CAD build for the part. Positions are in the model's coordinates, mm. A direction names the side the tool comes from. Round coordinates to 2 decimals unless told otherwise and drop trailing zeros. Order: outer loops, then holes, each group sorted by start corner. A loop starts at its lowest first (then second) coordinate and runs counter-clockwise, first axis right, second up. Notation, with made-up numbers: M 28,-13 L 44,-13 A15 ccw 44,10 Z; hole C 7.25,85 d2. An arc over 180 degrees is marked long. Answer as CSV lines item,"result". Start each with the question number.
```python
from build123d import *

# Parameters (mm, degrees)
SKETCH_1_R          = 1.6
SKETCH_1_R_2        = 2.1
EXTRUDE_2_DEPTH     = 3
SKETCH_2_R          = 2.1
CUT_EXTRUDE_1_DEPTH = 3
FILLET_1_R          = 3
CUT_EXTRUDE_2_DEPTH = 281.258651654


with BuildPart() as part:
    # 草图1 → 凸台-拉伸2 (new body)
    with BuildSketch(Plane.XY):
        Polygon((20.192307692, -5), (109.041451884, -5), (135.57179677, -50.951905284), (275.57179677, -50.951905284), (275.57179677, 31.048094716), (260.57179677, 31.048094716), (260.57179677, -38.951905284), (142.5, -38.951905284), (105, 26), (-105, 26), (-142.5, -38.951905284), (-260.57179677, -38.951905284), (-260.57179677, 31.048094716), (-275.57179677, 31.048094716), (-275.57179677, -50.951905284), (-135.57179677, -50.951905284), (-109.041451884, -5), (-20.192307692, -5), align=None)
        with Locations((-118.279056191, -9)):
            Circle(SKETCH_1_R, mode=Mode.SUBTRACT)
        with Locations((-128.279056191, -26.320508076)):
            Circle(SKETCH_1_R, mode=Mode.SUBTRACT)
        with Locations((-150.57179677, -44.951905284)):
            Circle(SKETCH_1_R, mode=Mode.SUBTRACT)
        with Locations((-180.57179677, -44.951905284)):
            Circle(SKETCH_1_R, mode=Mode.SUBTRACT)
        with Locations((-210.57179677, -44.951905284)):
            Circle(SKETCH_1_R, mode=Mode.SUBTRACT)
        with Locations((-268.07179677, -44.951905284)):
            Circle(SKETCH_1_R_2, mode=Mode.SUBTRACT)
        with Locations((-268.07179677, -24.951905284)):
            Circle(SKETCH_1_R_2, mode=Mode.SUBTRACT)
        with Locations((-268.07179677, 0.048094716)):
            Circle(SKETCH_1_R_2, mode=Mode.SUBTRACT)
        with Locations((-268.07179677, 25.048094716)):
            Circle(SKETCH_1_R_2, mode=Mode.SUBTRACT)
    extrude(amount=EXTRUDE_2_DEPTH)

    # 草图2 → 切除-拉伸1 (cut)
    with BuildSketch(Plane.XY.offset(3)):
        with Locations((-83, 21)):
            Circle(SKETCH_2_R)
        with Locations((-83, 1)):
            Circle(SKETCH_2_R)
        with Locations(Location((83, 1, 0), (0, 0, 180))):
            Circle(SKETCH_2_R)
        with Locations(Location((83, 21, 0), (0, 0, 180))):
            Circle(SKETCH_2_R)
    extrude(amount=-CUT_EXTRUDE_1_DEPTH, mode=Mode.SUBTRACT)

    # 圆角1
    fillet_1_edges = [part.edges().sort_by_distance(p)[0] for p in [
        (109.041451884, -5, 1.5),
        (-109.041451884, -5, 1.5),
        (135.57179677, -50.951905284, 1.5),
        (-135.57179677, -50.951905284, 1.5),
        (275.57179677, -50.951905284, 1.5),
        (275.57179677, 31.048094716, 1.5),
        (-275.57179677, -50.951905284, 1.5),
        (260.57179677, 31.048094716, 1.5),
        (-275.57179677, 31.048094716, 1.5),
        (260.57179677, -38.951905284, 1.5),
        (-260.57179677, 31.048094716, 1.5),
        (142.5, -38.951905284, 1.5),
        (-260.57179677, -38.951905284, 1.5),
        (105, 26, 1.5),
        (-142.5, -38.951905284, 1.5),
        (-105, 26, 1.5),
    ]]
    fillet(fillet_1_edges, radius=FILLET_1_R)

    # 草图3 → 切除-拉伸2 (cut, through all)
    with BuildSketch(Plane.XY.offset(3)):
        with BuildLine():
            Line((-59, 19), (-59, 4))
            ThreePointArc((-59, 4), (-63, 0), (-67, 4))
            Line((-67, 4), (-67, 19))
            ThreePointArc((-67, 19), (-63, 23), (-59, 19))
        make_face()
        with BuildLine():
            Line((-51.2, 19), (-51.2, 4))
            ThreePointArc((-51.2, 4), (-47.2, 0), (-43.2, 4))
            Line((-43.2, 4), (-43.2, 19))
            ThreePointArc((-43.2, 19), (-47.2, 23), (-51.2, 19))
        make_face()
        with BuildLine():
            Line((-35.4, 19), (-35.4, 4))
            ThreePointArc((-35.4, 4), (-31.4, 0), (-27.4, 4))
            Line((-27.4, 4), (-27.4, 19))
            ThreePointArc((-27.4, 19), (-31.4, 23), (-35.4, 19))
        make_face()
        with BuildLine():
            Line((-19.6, 19), (-19.6, 4))
            ThreePointArc((-19.6, 4), (-15.6, 0), (-11.6, 4))
            Line((-11.6, 4), (-11.6, 19))
            ThreePointArc((-11.6, 19), (-15.6, 23), (-19.6, 19))
        make_face()
        with BuildLine():
            Line((-3.8, 19), (-3.8, 4))
            ThreePointArc((-3.8, 4), (0.2, 0), (4.2, 4))
            Line((4.2, 4), (4.2, 19))
            ThreePointArc((4.2, 19), (0.2, 23), (-3.8, 19))
        make_face()
        with BuildLine():
            Line((12, 19), (12, 4))
            ThreePointArc((12, 4), (16, 0), (20, 4))
            Line((20, 4), (20, 19))
            ThreePointArc((20, 19), (16, 23), (12, 19))
        make_face()
        with BuildLine():
            Line((27.8, 19), (27.8, 4))
            ThreePointArc((27.8, 4), (31.8, 0), (35.8, 4))
            Line((35.8, 4), (35.8, 19))
            ThreePointArc((35.8, 19), (31.8, 23), (27.8, 19))
        make_face()
        with BuildLine():
            Line((43.6, 19), (43.6, 4))
            ThreePointArc((43.6, 4), (47.6, 0), (51.6, 4))
            Line((51.6, 4), (51.6, 19))
            ThreePointArc((51.6, 19), (47.6, 23), (43.6, 19))
        make_face()
        with BuildLine():
            Line((59.4, 19), (59.4, 4))
            ThreePointArc((59.4, 4), (63.4, 0), (67.4, 4))
            Line((67.4, 4), (67.4, 19))
            ThreePointArc((67.4, 19), (63.4, 23), (59.4, 19))
        make_face()
    extrude(amount=-CUT_EXTRUDE_2_DEPTH, mode=Mode.SUBTRACT)


solid = part.part
```
Q1. Mould opens along X. For faces 1 (the flat face through (124, -6.91, 1.48)), 2 (the flat face through (-122.48, -28.28, 1.48)), 3 (the flat face through (19, -1, 3)) say: +X half, -X half, draft (parallel to the pull), parting line (faces both ways), or undercut.
Q2. Band-saw the part on A-A, the plane y = 11. Count the separate pieces of the cut face and the enclosed holes in it, then the cut area to 3 significant figures.
Q3. Band-saw the part on B-B, the plane x = -235. Write the cut outline in (y, z), then the cut area to 3 significant figures.
Q4. Tool access for faces 4 (the flat face through (122.133, -27.675, 1.479)), 5 (the flat face through (19, -1, 0)), 6 (the flat face through (-123.5, -6.04, 1.48)): list every direction of +Z, -Z, +X, -X, +Y, -Y with a clear straight run to the whole face (end or side of a thin tool).
Q5. Probe line 1 along X through (y, z) = (24.5, 1.25); line 2 along Y through (x, z) = (-83, 2.2); line 3 along Y through (x, z) = (-150.5, 0.45). List the from-to ranges inside material, lowest first. Write a range as from..to.
Q6. Drop flat-ended pins along their axis: P1, Ø1, axis at x = 2.5, z = 1.5, coming from the -Y side; P2, Ø3.5, axis at x = -83, y = 21, coming from the +Z side. Give the stop position or say it passes through.
Answer:
1,face 1,"undercut"
1,face 2,"undercut"
1,face 3,"draft"
2,separate pieces,"12"
2,enclosed holes,"0"
2,area,"556 mm^2"
3,outline,"M -50.95,0 L -38.95,0 L -38.95,3 L -50.95,3 Z"
3,area,"36.0 mm^2"
4,face 4,"+Z, -Z, -Y"
4,face 5,"-Z, +X, -X, +Y, -Y"
4,face 6,"+Z, -Z, +Y"
5,line 1,"x = -275.57..-270.1, -266.04..-260.57, -105.87..105.87, 260.57..275.57"
5,line 2,"y = -5..-1.1, 3.1..18.9, 23.1..26"
5,line 3,"y = -50.95..-46.55, -43.35..-38.95"
6,P1,"stops at y = -5"
6,P2,"passes through"
